Here's how the part is built. I have some questions about the finished solid (model axes, mm). Face numbers are marked on the shaded views. Give positions to 0.01 mm unless a question says otherwise; leave off trailing zeros. Order: outer loops, then holes, each group sorted by start corner. A loop starts at its lowest first (then second) coordinate and runs counter-clockwise, first axis right, second up. Notation, with made-up numbers: M -6,76 L 50,76 A32 ccw 50,112 Z; hole C -6,-31 d2. An arc over 180 degrees is marked long. One line per item, written item: value. Start each with the question number.
Autodesk Inventor part; units mm, degrees
ref_plane "YZ Plane" through (0, 0, 0) normal (1, 0, 0) x (0, 1, 0)
ref_plane "XZ Plane" through (0, 0, 0) normal (0, 1, 0) x (-1, 0, 0)
ref_plane "XY Plane" through (0, 0, 0) normal (0, 0, 1) x (1, 0, 0)
sketch "Sketch1" plane through (0, 0, 0) normal (0, 1, 0) x (-1, 0, 0)
  circle A0 centre (0, 0) radius 11.25
  circle A1 centre (0, 0) radius 14.25
  circle A2 centre (0, 0) radius 30
  circle A3 centre (0, 0) radius 6.75
  dimension "d0" = 22.5
  dimension "d1" = 28.5
  dimension "d2" = 60
  dimension "d3" = 13.5
extrude "Extrusion1" add sketch "Sketch1" along normal blind 4.5 contours A0 | A1
sketch "Sketch2" plane through (0, 4.5, 0) normal (0, 1, 0) x (1, 0, 0)
  circle A0 centre (0, 0) radius 14.25
  circle A1 centre (0, 0) radius 11.25
  dimension "d6" = 22.5
extrude "Extrusion2" add sketch "Sketch2" along normal blind 8
sketch "Sketch3" plane through (0, 12.5, 0) normal (0, 1, 0) x (1, 0, 0)
  circle A0 centre (0, 0) radius 14.25
  circle A1 centre (0, 0) radius 25.25
  dimension "d9" = 50.5
extrude "Extrusion3" add sketch "Sketch3" against normal blind 3
chamfer "Chamfer2" distance 4.5 angle 45 1 edges at (6.75, 4.5, 0)
fillet "Fillet1" radius 5 1 edges at (14.25, 0, 0)
fillet "Fillet2" radius 2 1 edges at (-14.25, 9.5, 0)
fillet "Fillet3" radius 1 1 edges at (-25.25, 9.5, 0)
sketch "Sketch5" plane through (0, 9.5, 0) normal (0, -1, 0) x (1, 0, 0)
  circle A0 centre (0, 0) radius 16.25
  circle A1 centre (-20, 0) radius 1.5
  circle A2 centre (-20, 0) radius 3.75
  circle A3 centre (20, 0) radius 1.5
  circle A4 centre (0, -20) radius 1.5
  circle A5 centre (0, 20) radius 1.5
  dimension "d21" = 3
  dimension "d22" = 20
  dimension "d23" = 3
  dimension "d24" = 20
  dimension "d25" = 3
  dimension "d26" = 20
  dimension "d27" = 3
  dimension "d28" = 20
extrude "Extrusion4" cut sketch "Sketch5" against normal blind 11 contours A1 | A3 | A4 | A5
sketch "Sketch6" plane through (0, 0, 0) normal (0, -1, 0) x (1, 0, 0)
  circle A0 centre (0, 0) radius 9.25
  circle A1 centre (0, 0) radius 18.9593
extrude "Extrusion5" cut sketch "Sketch6" against normal blind 2.5 contours A0 | A1
sketch "Sketch7" plane through (0, 2.5, 0) normal (0, -1, 0) x (1, 0, 0)
  circle A0 centre (0, 0) radius 13.5801
  circle A1 centre (0, 0) radius 9.25
fillet "Fillet4" radius 3 2 edges at (0, 2.5, 13.5801) (0, 2.5, -13.5801)
properties part number "supportoCuscinettoAlto"
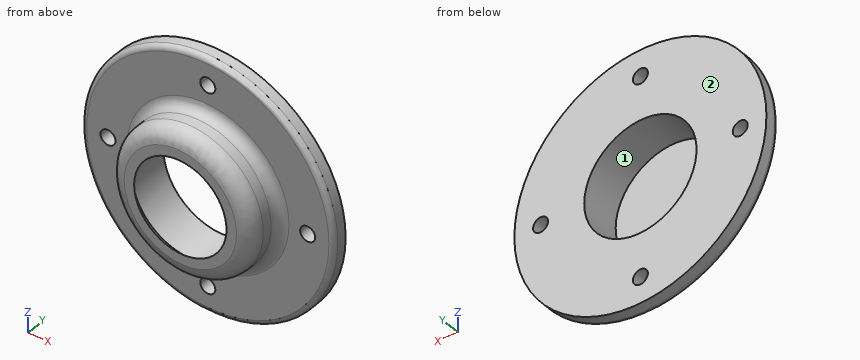
Item 1: We'd pull the mould along Z, two halves only. Please class the marked faces 1 and 2: +Z half, -Z half, draft (parallel to the pull), parting line (faces both ways), or undercut.
Item 2: I want a section at A-A on y = 11.5. Write out the boundary of the cut face in (x, z), plus the area to 3 significant figures.
Item 3: Please list where these lines run through material, in increasing order: probe 1 along Z at (x, y) = (0, 10.9); probe 2 along X at (y, z) = (4.5, -9); probe 3 along Y at (x, z) = (-16, -2.5). Write a range as [from, to].
Item 4: I want a section at B-B on y = 6.5. Write out the boundary of the cut face in (x, z).
Item 5: Will these pins go through, and if not, where does the flat tip stop? P1, Ø2.5, axis at x = -20, z = 0, coming from the -Y side; P2, Ø3, axis at x = -9, y = 9.5, coming from the +Z side; P3, Ø3, axis at y = 10.5, z = 12, coming from the +X side; P4, Ø5, axis at x = 15, z = -16, coming from the -Y side.
Answer below:
1. face 1: undercut
1. face 2: draft
2. outline: C 0,0 d50.5; hole C -20,0 d3; hole C 0,0 d22.5; hole C 0,-20 d3; hole C 0,20 d3; hole C 20,0 d3
2. area: 1,580 mm²
3. probe 1: z = [-25.25, -21.5], [-18.5, -11.25], [11.25, 18.5], [21.5, 25.25]
3. probe 2: x = [-10.83, -6.75], [6.75, 10.83]
3. probe 3: y = [9.5, 12.5]
4. outline: C 0,0 d28.5; hole C 0,0 d22.5
5. P1: passes through
5. P2: stops at z = 24.02
5. P3: stops at x = 22.96
5. P4: stops at y = 9.5
